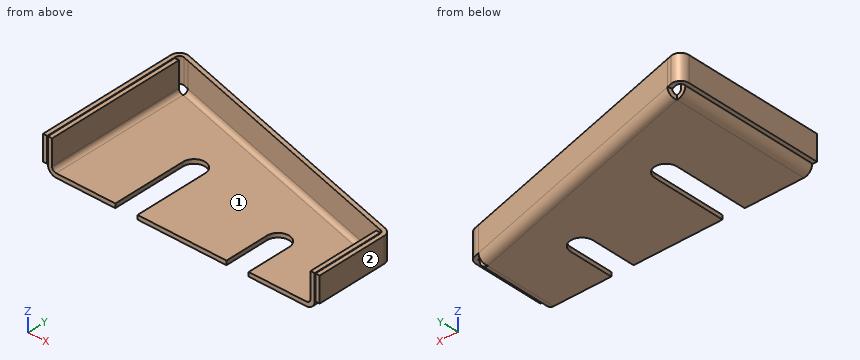
from build123d import *

# Parameters (mm, degrees)
PAD_DEPTH            = 24
THICKNESS_T          = -3
FILLET_R             = 3
FILLET001_R          = 6
POCKET_DEPTH         = 24.001
SKETCH003_W          = 3
SKETCH003_H          = 18
SKETCH005_W          = 3
SKETCH005_H          = 18
POCKET001_DEPTH      = 0.001
POCKET001_DEPTH_BACK = 24.001


with BuildPart() as part:
    # Sketch (on XY_Plane of Origin) → Pad (new body)
    with BuildSketch(Plane.XY):
        Polygon((-6, 0), (186, 0), (186, 56.373107), (-6, 107.819352), align=None)
    extrude(amount=PAD_DEPTH)

    # Thickness
    thickness_openings = [part.faces().sort_by_distance(p)[0] for p in [
        (79.973475, 42.391415, 24),
        (90, 0, 12),
    ]]
    offset(amount=THICKNESS_T, openings=thickness_openings, kind=Kind.INTERSECTION)

    # Fillet
    fillet_edges = [part.edges().sort_by_distance(p)[0] for p in [
        (-3, 51.954838, 3),
        (183, 27.035563, 3),
        (90, 78.990401, 3),
    ]]
    fillet(fillet_edges, radius=FILLET_R)

    # Fillet001
    fillet001_edges = [part.edges().sort_by_distance(p)[0] for p in [
        (90, 82.09623, 0),
        (-6, 53.909676, 0),
        (186, 28.186554, 0),
    ]]
    fillet(fillet001_edges, radius=FILLET001_R)

    # Sketch001 (on Face5 of Fillet001) → Pocket (cut, through all)
    with BuildSketch(Plane(origin=(0, 0, 0), x_dir=(1, 0, 0), z_dir=(0, 0, -1))):
        Polygon((186, -51.769145), (186, -56.373107), (181.552914, -57.5647), (180, -51.769145), align=None)
        Polygon((0, -100), (1.552914, -105.795555), (-6, -107.819352), (-6, -100), align=None)
    extrude(amount=-POCKET_DEPTH, mode=Mode.SUBTRACT)

    # AdditivePipe: sweep along a path in Sketch002
    with BuildLine(Plane.XY.offset(24)) as additivepipe_path:
        Line((0.776457, 102.897777), (-2.723543, 103.8356))
        ThreePointArc((-2.723543, 103.8356), (-5.326284, 103.317882), (-6.5, 100.937822))
        Line((-6.5, 100.937822), (-6.5, 0))
    # Sketch003 (on Face18 of Pocket) → AdditivePipe (sweep)
    with BuildSketch(Plane(origin=(-25, 6.69873, 0), x_dir=(-0.258819, -0.965926, 0), z_dir=(-0.965926, 0.258819, 0))):
        with Locations((-101.092583, 15)):
            Rectangle(SKETCH003_W, SKETCH003_H)
    sweep(path=additivepipe_path.line)

    # AdditivePipe001: sweep along a path in Sketch006
    with BuildLine(Plane.XY.offset(24)) as additivepipe001_path:
        Line((186.5, 0), (186.5, 50.831323))
        ThreePointArc((186.5, 50.831323), (185.88006, 52.657607), (184.276457, 53.729101))
        Line((184.276457, 53.729101), (180.776457, 54.666923))
    # Sketch005 (on Face2 of AdditivePipe) → AdditivePipe001 (sweep)
    with BuildSketch(Plane(origin=(155, -41.532125, 0), x_dir=(0.258819, 0.965926, 0), z_dir=(0.965926, -0.258819, 0))):
        with Locations((101.092583, 15)):
            Rectangle(SKETCH005_W, SKETCH005_H)
    sweep(path=additivepipe001_path.line)

    # Sketch004 (on XY_Plane of Origin) → Pocket001 (cut, two sides)
    with BuildSketch(Plane.XY) as pocket001_sk:
        with BuildLine():
            ThreePointArc((42.5, 0), (50.5, -8), (58.5, 0))
            Line((58.5, 0), (58.5, 53.339728))
            ThreePointArc((58.5, 53.339728), (50.5, 61.339728), (42.5, 53.339728))
            Line((42.5, 0), (42.5, 53.339728))
        make_face()
        with BuildLine():
            ThreePointArc((138.5, 31.903793), (130.5, 39.903793), (122.5, 31.903793))
            Line((122.5, 31.903793), (122.5, 0))
            ThreePointArc((122.5, 0), (130.5, -8), (138.5, 0))
            Line((138.5, 31.903793), (138.5, 0))
        make_face()
    extrude(amount=-POCKET001_DEPTH, mode=Mode.SUBTRACT)
    extrude(pocket001_sk.sketch, amount=POCKET001_DEPTH_BACK, mode=Mode.SUBTRACT)


solid = part.part
Could you check a few things on this model? Use its own coordinates, in mm. Face numbers are marked on the shaded views. A direction names the side the tool comes from. Give positions to 0.01 mm unless a question says otherwise; leave off trailing zeros. Order: outer loops, then holes, each group sorted by start corner. A loop starts at its lowest first (then second) coordinate and runs counter-clockwise, first axis right, second up.
1. Will these pins go through, and if not, where does the flat tip stop? P1, Ø3, axis at x = 30.5, z = 6.5, coming from the -Y side; P2, Ø1.5, axis at y = 17.5, z = 2, coming from the -X side; P3, Ø10, axis at x = 68, z = 13, coming from the +Y side.
2. For the marked faces 1 and 2, which set-ups out of +Z, -Z, +X, -X, +Y, -Y let a thin tool reach every point of the face, with its end or its side?
3. I need wall thicknesses on L1, parallel to X at y = 30, z = 14.25; L2, parallel to X at y = 25, z = 1.25; L3, parallel to Z at x = 18.5, y = 14.5. Which ranges of each line are inside material? Lowest first, please.
4. Suppose I cut it at B-B (y = 16.5). List the corners of the cut face in (x, z) for me.
5. Suppose I cut it at A-A (z = 14). List the corners of the cut face in (x, y) for me, plus the area to 3 significant figures.
6. Suppose I cut it at C-C (y = 48). List the corners of the cut face in (x, z) for me, plus the area to 3 significant figures.
Solved:
1. P1: stops at y = 94.53
1. P2: stops at x = -5.04
1. P3: stops at y = 89.33
2. face 1: +Z, -Y
2. face 2: +Z, -Z, +X, +Y, -Y
3. L1: x = -9.5 to -6.5, -6 to -3, 183 to 186, 186.5 to 189.5
3. L2: x = -3.67 to 42.5, 58.5 to 122.5, 138.5 to 183.67
3. L3: z = 0 to 3
4. outline: (-9.5, 6) - (-6.5, 6) - (-6.5, 24) - (-9.5, 24) - close; (-6, 6) arc R6 ccw to (0, 0) - (42.5, 0) - (42.5, 3) - (0, 3) arc R3 cw to (-3, 6) - (-3, 24) - (-6, 24) - close; (58.5, 0) - (122.5, 0) - (122.5, 3) - (58.5, 3) - close; (138.5, 0) - (180, 0) arc R6 ccw to (186, 6) - (186, 24) - (183, 24) - (183, 6) arc R3 cw to (180, 3) - (138.5, 3) - close; (186.5, 6) - (189.5, 6) - (189.5, 24) - (186.5, 24) - close
5. outline: (-9.5, 0) - (-6.5, 0) - (-6.5, 100.94) arc R3 cw to (-2.72, 103.84) - (0.78, 102.9) - (184.28, 53.73) arc R3 cw to (186.5, 50.83) - (186.5, 0) - (189.5, 0) - (189.5, 50.83) arc R6 ccw to (185.05, 56.63) - (1.55, 105.8) - (-1.95, 106.73) arc R6 ccw to (-9.5, 100.94) - close; (-6, 0) - (-3, 0) - (-3, 100) - (-6, 100) - close; (183, 0) - (186, 0) - (186, 51.77) - (183, 51.77) - close
5. area: 1,530 mm2
6. outline: (-9.5, 6) - (-6.5, 6) - (-6.5, 24) - (-9.5, 24) - close; (-6, 6) arc R6 ccw to (0, 0) - (42.5, 0) - (42.5, 3) - (0, 3) arc R3 cw to (-3, 6) - (-3, 24) - (-6, 24) - close; (58.5, 0) - (180, 0) arc R6 ccw to (186, 6) - (186, 24) - (183, 24) - (183, 6) arc R3 cw to (180, 3) - (58.5, 3) - close; (186.5, 6) - (189.5, 6) - (189.5, 24) - (186.5, 24) - close
6. area: 750 mm2
